The drawing under review shows one solid part. Ordinate dimensions are in mm from its lowest x, y, z. A direction names the side the tool comes from. Coordinates: 2 decimals unless noted, no trailing zeros. Loops run counter-clockwise (first coordinate to the right, second up) from the corner with the lowest first, then second, coordinate; pieces in that order, holes last. Notation, with made-up numbers: (42.25, 3) - (58.25, 3) arc R16 ccw to (58.25, 23) - close; hole circle Ø6 at (61.5, 82). An arc over 180 degrees is marked (long way). Answer as a JSON object with one key per item and string values. Group by question number.
Item 1: Tool access review of the marked faces 1 and 2: name each direction out of +Z, -Z, +X, -X, +Y, -Y from which nothing blocks a thin tool from reaching the whole face with its end or side.
Item 2: To check wall thickness, follow line 1 (X direction, y = 14.6, z = 7); line 2 (Z direction, x = 1, y = 8.25); line 3 (Z direction, x = 5, y = 15.15). State the ranges of each line that lie inside material, in increasing order.
Item 3: We need section B-B (x = 5). Give the boundary of the cut face in (y, z), then the cut area to 3 significant figures.
Item 4: Mouldability with a two-part tool opening along Z and no side actions: class the marked faces 3, 4 and 5 as released by +Z, released by -Z, zero draft, split by the parting line, or undercut.
Item 5: We need section A-A (y = 7). Give the boundary of the cut face in (x, z), then the cut area to 3 significant figures.
Item 6: Clearance check with flat-ended pins moving along their axes: pin 1 (6 mm diameter, centred on y = 6, z = 8.5, fed in from +X); pin 2 (5 mm diameter, centred on x = 9.5, z = 8.5, fed in from -Y). State where each tip first meets the part, or that it passes through.
Item 7: We need section D-D (x = 7.5). Give the boundary of the cut face in (y, z), then the cut area to 3 significant figures.
Item 8: We need section C-C (z = 7). Give the boundary of the cut face in (x, y).
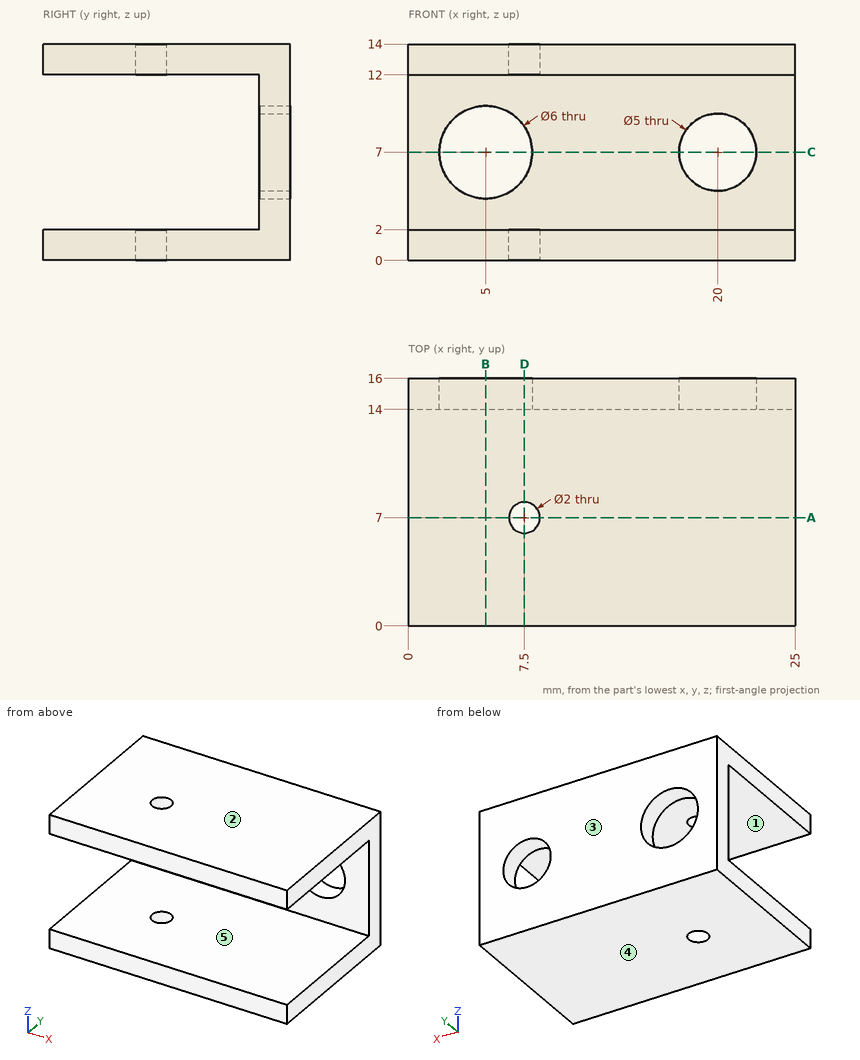
Check sheet entries:
{
 "1": {"face 1": "+X, -X, -Y", "face 2": "+Z, +X, -X, +Y, -Y"},
 "2": {"line 1": "x = 0 to 2, 8 to 17.5, 22.5 to 25", "line 2": "z = 0 to 2, 12 to 14", "line 3": "z = 0 to 4, 10 to 14"},
 "3": {"outline": "(0, 0) - (16, 0) - (16, 4) - (14, 4) - (14, 2) - (0, 2) - close; (0, 12) - (14, 12) - (14, 10) - (16, 10) - (16, 14) - (0, 14) - close", "area": "72.0 mm2"},
 "4": {"face 3": "zero draft", "face 4": "released by -Z", "face 5": "undercut"},
 "5": {"outline": "(0, 0) - (6.5, 0) - (6.5, 2) - (0, 2) - close; (0, 12) - (6.5, 12) - (6.5, 14) - (0, 14) - close; (8.5, 0) - (25, 0) - (25, 2) - (8.5, 2) - close; (8.5, 12) - (25, 12) - (25, 14) - (8.5, 14) - close", "area": "92.0 mm2"},
 "6": {"pin 1": "passes through", "pin 2": "stops at y = 14"},
 "7": {"outline": "(0, 0) - (6, 0) - (6, 2) - (0, 2) - close; (0, 12) - (6, 12) - (6, 14) - (0, 14) - close; (8, 0) - (16, 0) - (16, 5.34) - (14, 5.34) - (14, 2) - (8, 2) - close; (8, 12) - (14, 12) - (14, 8.66) - (16, 8.66) - (16, 14) - (8, 14) - close", "area": "69.4 mm2"},
 "8": {"outline": "(0, 14) - (2, 14) - (2, 16) - (0, 16) - close; (8, 14) - (17.5, 14) - (17.5, 16) - (8, 16) - close; (22.5, 14) - (25, 14) - (25, 16) - (22.5, 16) - close"}
}
